```python
from build123d import *

# Parameters (mm, degrees)
SKETCH1_R                 = 7.62
BOSS_EXTRUDE1_DEPTH       = 6.35
F_6_32_TAPPED_HOLE1_D     = 2.7051
F_6_32_TAPPED_HOLE1_DEPTH = 9.398
F_6_32_TAPPED_HOLE1_TIP   = 0.81269403


with BuildPart() as part:
    # Sketch1 → Boss-Extrude1 (new body)
    with BuildSketch(Plane(origin=(0, 0, 0), x_dir=(1, 0, 0), z_dir=(0, 1, 0))):
        with Locations(Location((0, 0, 0), (0, 0, 270))):
            Circle(SKETCH1_R)
    extrude(amount=-BOSS_EXTRUDE1_DEPTH)

    # Sketch3 one side → Revolve1 (revolve)
    with BuildSketch(Plane.XY, mode=Mode.PRIVATE) as revolve1_sk:
        with BuildLine():
            Line((0, 117.206637485), (0, 115.174637485))
            Line((0, 115.174637485), (0, 0))
            Line((0, 0), (11.39145745, 0))
            Line((11.39145745, 0), (1.011976427, 116.280968605))
            ThreePointArc((1.011976427, 116.280968605), (0.685740324, 116.940314889), (0, 117.206637485))
        make_face()
    revolve(revolve1_sk.sketch.rotate(Axis((0, 0, 0), (0, 1, 0)), 90), axis=Axis((0, 0, 0), (0, 1, 0)))

    # 6-32 Tapped Hole1
    with Locations(Plane.XZ.offset(6.35)):
        with Locations((0, 0)):
            Hole(F_6_32_TAPPED_HOLE1_D / 2, depth=F_6_32_TAPPED_HOLE1_DEPTH)
            with Locations((0, 0, -(F_6_32_TAPPED_HOLE1_DEPTH + F_6_32_TAPPED_HOLE1_TIP / 2))):  # 118° drill point
                Cone(0, F_6_32_TAPPED_HOLE1_D / 2, F_6_32_TAPPED_HOLE1_TIP, mode=Mode.SUBTRACT)


solid = part.part
```
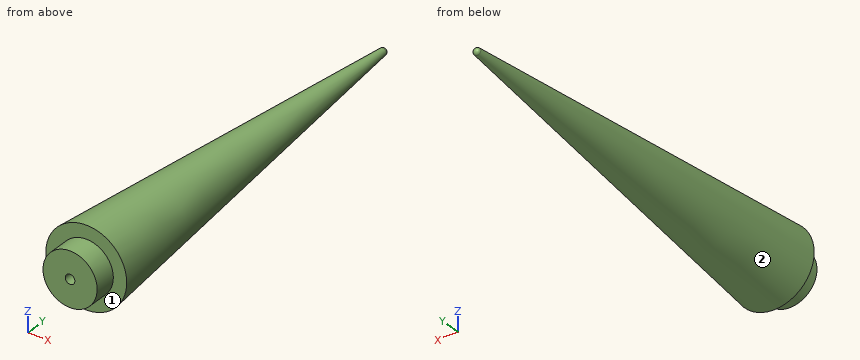
Can you work these out from the model? Positions are in its coordinate system, mm. Face numbers are marked on the shaded views. A direction names the side the tool comes from. Give positions to 0.01 mm unless a question says otherwise; leave off trailing zeros. Loops run counter-clockwise (first coordinate to the right, second up) from the corner with the lowest first, then second, coordinate; pieces in that order, holes last. Notation, with made-up numbers: M -37.5,35.25 L -11.5,35.25 A25 ccw -11.5,64.25 Z; hole C 1.25,56 d8. An arc over 180 degrees is marked long. Answer in a Markdown table with one row per item.
1. For pin 1 Ø2 at (x, z) = (4.5, 8.5) entering from -Y; pin 2 Ø1.5 at (x, z) = (8.5, 9) entering from -Y; pin 3 Ø3 at (y, z) = (78.5, 2) entering from -X; pin 4 Ø8 at (x, z) = (8.5, 5) entering from -Y, each with a flat end and sliding along its axis, tell me the tip position at first contact or that it passes through.
Taken from the geometry:
| item | result |
|---|---|
| pin 1 | stops at y = 0 |
| pin 2 | passes through |
| pin 3 | stops at x = -4.4 |
| pin 4 | stops at y = -6.35 |
2. Suppose I cut it at B-B on y = 45. Write out the boundary of the cut face in (x, z).
Taken from the geometry:
| item | result |
|---|---|
| outline | C 0,0 d14.75 |
3. Which directions (+Z, -Z, +X, -X, +Y, -Y) give clear straight access to the entire face, cutting with the end or side of a thin tool? Please do the marked faces 1 and 2.
Taken from the geometry:
| item | result |
|---|---|
| face 1 | -Y |
| face 2 | +Y |
4. Suppose I cut it at A-A on y = 94. Write out the boundary of the cut face in (x, z), plus the area to 3 significant figures.
Taken from the geometry:
| item | result |
|---|---|
| outline | C 0,0 d6 |
| area | 28.3 mm² |
5. If I drill on line 1 along X through (y, z) = (-1.5, 0); line 2 along X through (y, z) = (70, -2.5); line 3 along X through (y, z) = (23.5, -1.75), over which ranges is the centre line in solid material (lowest first)?
Taken from the geometry:
| item | result |
|---|---|
| line 1 | x = -7.62 to -1.35, 1.35 to 7.62 |
| line 2 | x = -4.49 to 4.49 |
| line 3 | x = -9.13 to 9.13 |
